The drawing under review shows one solid part. Ordinate dimensions are in mm from its lowest x, y, z. A direction names the side the tool comes from. Coordinates: 2 decimals unless noted, no trailing zeros. Loops run counter-clockwise (first coordinate to the right, second up) from the corner with the lowest first, then second, coordinate; pieces in that order, holes last. Notation, with made-up numbers: M 62,-31.5 L 87,-31.5 A18 ccw 87,-8.5 Z; hole C 76,59 d8. An arc over 180 degrees is marked long. Answer as a JSON object with one key per item and string values. Group by question number.
1. Consider section D-D (z = 150.5). State the section outline as (x, y) points, then the cut area to 3 significant figures.
2. Machinability: for the marked faces 1 and 2, which of the approach directions +Z, -Z, +X, -X, +Y, -Y give a long, thin tool a straight path to every point of the face, cutting with its end or side? Answer none if there is none.
3. Insertion check: pin 1 (10 mm diameter, centred on x = 53, z = 35.5, fed in from +Y); pin 2 (1 mm diameter, centred on y = 26, z = 114, fed in from +X); pin 3 (1 mm diameter, centred on x = 35.5, z = 177.5, fed in from -Y); pin 4 (2 mm diameter, centred on y = 52.5, z = 25.5, fed in from +X). Each pin has a flat end and moves straight along its axis. Give the tip position at first contact, or say it passes through.
4. To check wall thickness, follow probe 1 along Y at (x, z) = (33.5, 50.5); probe 2 along Z at (x, y) = (27, 40); probe 3 along X at (y, z) = (10, 10) (1 decimal). State the ranges of each line that lie inside material, in increasing order.
5. Consider section A-A (z = 44.5). State the section outline as (x, y) points.
6. Consider section C-C (x = 30.5). State the section outline as (y, z) points, then the cut area to 3 significant figures.
7. Consider section B-B (y = 28.5). State the section outline as (x, z) points, then the cut area to 3 significant figures.
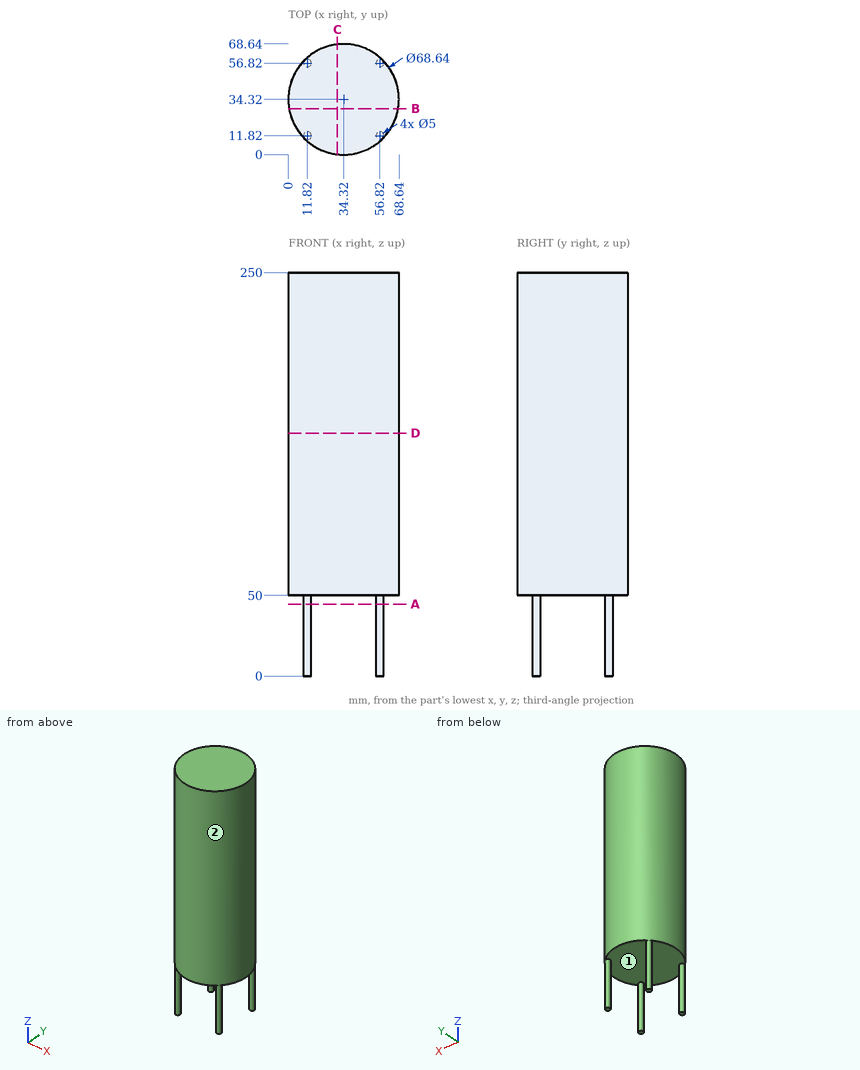
Findings below:
{
 "1": {"outline": "C 34.32,34.32 d68.64", "area": "3,700 mm^2"},
 "2": {"face 1": "-Z", "face 2": "+Z, -Z"},
 "3": {"pin 1": "stops at y = 59.32", "pin 2": "stops at x = 67.74", "pin 3": "stops at y = 0.01", "pin 4": "passes through"},
 "4": {"probe 1": "y = 0.01 to 68.63", "probe 2": "z = 50 to 250", "probe 3": "x = 10.1 to 13.5, 55.1 to 58.5"},
 "5": {"outline": "C 11.82,11.82 d5; C 11.82,56.82 d5; C 56.82,11.82 d5; C 56.82,56.82 d5"},
 "6": {"outline": "M 0.21,50 L 68.43,50 L 68.43,250 L 0.21,250 Z", "area": "13,600 mm^2"},
 "7": {"outline": "M 0.5,50 L 68.14,50 L 68.14,250 L 0.5,250 Z", "area": "13,500 mm^2"}
}
